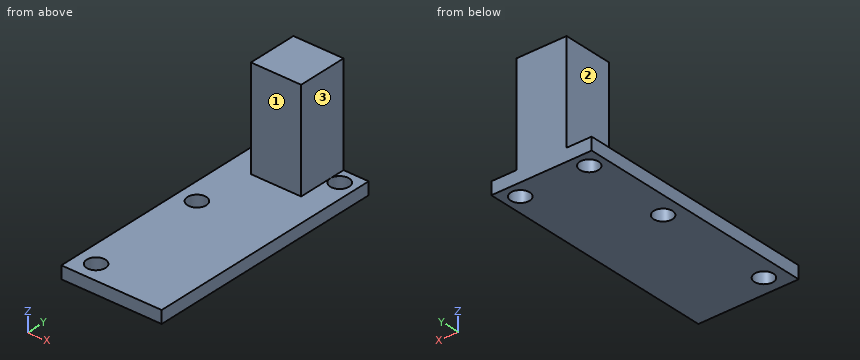
Solid Edge part; units mm, degrees
sketch "Sketch1" plane through (0, 0, 0) normal (0, 0, 1) x (1, 0, 0)
  line L0 (0, 0) -> (16, 0)
  line L1 (16, 0) -> (16, 39)
  line L2 (16, 39) -> (0, 39)
  line L3 (0, 39) -> (0, 0)
  dimension "D1" = 16
extrude "Protrusion1" add sketch "Sketch1" along normal blind 2
sketch "Sketch2" plane through (8, 19.5, 2) normal (0, 0, 1) x (1, 0, 0)
  circle A0 centre (-5, 2.5) radius 1.5
  circle A1 centre (-5.5, 17) radius 1.5
  circle A2 centre (5.5, 17) radius 1.5
  circle A3 centre (-5, -16.5) radius 1.5
  dimension "D1" = 5
  dimension "D2" = 5.5
  dimension "D3" = 5.5
extrude "Cutout1" cut sketch "Sketch2" against normal through all
sketch "Sketch3" plane through (8, 19.5, 2) normal (0, 0, 1) x (1, 0, 0)
  line L0 (-4, 11.5) -> (4, 11.5)
  line L1 (4, 11.5) -> (4, 19.5)
  line L2 (4, 19.5) -> (-4, 19.5)
  line L3 (-4, 19.5) -> (-4, 11.5)
  dimension "D1" = 4
  dimension "D2" = 4
extrude "ExtrudedProtrusion_2" add sketch "Sketch3" along normal blind 16
Part model, mm, in its own coordinate system. Face numbers are marked on the shaded views. A direction names the side the tool comes from. Round coordinates to 2 decimals unless told otherwise and drop trailing zeros. Write each loop counter-clockwise with the first axis right and the second up, starting at its lowest first coordinate (ties: lowest second). Pieces come first, ordered by that corner, then holes. Notation, with made-up numbers: M -17.75,25 L 23.25,25 A23 cw 23.25,38 Z; hole C 23,75.25 d4. An arc over 180 degrees is marked long. Answer as CSV lines item,"result". Start each with the question number.
1) Band-saw the part on B-B (x = 13). List the corners of the cut face in (y, z).
2) Band-saw the part on A-A (y = 3). List the corners of the cut face in (x, z), then the cut area to 3 significant figures.
3) Drop flat-ended pins along their axis: pin 1 (2.5 mm diameter, centred on x = 8.5, z = 12, fed in from -Y); pin 2 (6.5 mm diameter, centred on y = 36.5, z = 11.5, fed in from -X); pin 3 (2.5 mm diameter, centred on x = 2.5, y = 36.5, fed in from -Z); pin 4 (8 mm diameter, centred on x = 11, y = 13.5, fed in from +Z). Give the stop position or say it passes through.
4) Band-saw the part on C-C (x = 3). List the corners of the cut face in (y, z).
5) Which spindle directions (+Z, -Z, +X, -X, +Y, -Y) get a long thin tool onto all of the face, cutting with end or side? Do the marked faces 1, 2 and 3. Say none if no direction does.
6) Drill centre lines: L1, parallel to Y at x = 3, z = 0.7; L2, parallel to Y at x = 13.5, z = 1.15; L3, parallel to Z at x = 12.75, y = 7. Where is each one in solid material? Low to high.
7) Band-saw the part on D-D (z = 4). List the corners of the cut face in (x, y), then the cut area to 3 significant figures.
Worked out:
1,outline,"M 0,0 L 35.09,0 L 35.09,2 L 0,2 Z; M 37.91,0 L 39,0 L 39,2 L 37.91,2 Z"
2,outline,"M 0,0 L 1.5,0 L 1.5,2 L 0,2 Z; M 4.5,0 L 16,0 L 16,2 L 4.5,2 Z"
2,area,"26.0 mm²"
3,pin 1,"y = 31"
3,pin 2,"x = 4"
3,pin 3,"through"
3,pin 4,"z = 2"
4,outline,"M 0,0 L 1.5,0 L 1.5,2 L 0,2 Z; M 4.5,0 L 20.5,0 L 20.5,2 L 4.5,2 Z; M 23.5,0 L 35.09,0 L 35.09,2 L 23.5,2 Z; M 37.91,0 L 39,0 L 39,2 L 37.91,2 Z"
5,face 1,"+Z, +X, -X, -Y"
5,face 2,"+Z, -X, +Y, -Y"
5,face 3,"+Z, +X, +Y, -Y"
6,L1,"0 to 1.5, 4.5 to 20.5, 23.5 to 35.09, 37.91 to 39"
6,L2,"0 to 35, 38 to 39"
6,L3,"0 to 2"
7,outline,"M 4,31 L 12,31 L 12,39 L 4,39 Z"
7,area,"64.0 mm²"
